from build123d import *

# Parameters (mm, degrees)
F0_W     = 62.186198
F0_H     = 153.296209
F1_DEPTH = 45.974
F2_R     = 22.70519
F3_DEPTH = 32.258
F5_DEPTH = 24.384


with BuildPart() as f1:
    # F0 (on Front) → F1 (new body)
    with BuildSketch(Plane.XZ):
        with Locations((1.59081, -0.433858)):
            Rectangle(F0_W, F0_H)
    extrude(amount=F1_DEPTH)

    # F2 (on face) → F3 (join)
    with BuildSketch(Plane.XZ.offset(45.974)):
        Circle(F2_R)
    extrude(amount=F3_DEPTH)

    # F4 (on Right) → F5 (cut, symmetric)
    with BuildSketch(Plane.YZ):
        Polygon((-53.611651, -25.310941), (-78.850865, 22.487216), (-78.627512, -25.310941), align=None)
    extrude(amount=F5_DEPTH, both=True, mode=Mode.SUBTRACT)


solid = f1.part
Build history of the part. All positions in model axes, mm. A direction names the side the tool comes from. Coordinates: 2 decimals unless noted, no trailing zeros. Order: outer loops, then holes, each group sorted by start corner. A loop starts at its lowest first (then second) coordinate and runs counter-clockwise, first axis right, second up. Notation, with made-up numbers: (-23.5, 18.25) - (-4.5, 18.25) arc R22 cw to (-4.5, 24.25) - close; hole circle Ø8 at (85, -38). An arc over 180 degrees is marked (long way). Write item = value, one per line. Start each with the question number.
1) Saw through at D-D on x = 26.5. Write the cut outline in (y, z), then the cut area to 3 significant figures.
2) Saw through at A-A on x = 0. Write the cut outline in (y, z).
3) 3-axis set-ups, long thin cutter, end or side, ignore diameter. For faces 1 (the face through (-2.96, -58.29, 22.51)), 2 (the face through (0.32, -66.45, -1)): which of +Z, -Z, +X, -X, +Y, -Y reach the whole face in a straight line?
4) Saw through at B-B on z = -1.5. Write the cut outline in (x, y), then the cut area to 3 significant figures.
5) Wall check: line 1 along Y through (x, z) = (9.5, 43); line 2 along X through (y, z) = (-53.5, 10.5); line 3 along Z through (x, y) = (4.5, -52.5). Give the ranges that are in metal, low to high. Write a range as from..to.
6) Flat gauge pins, fed straight in: pin 1 Ø4 at (x, y) = (-2.5, -65.5) entering from +Z; pin 2 Ø10 at (x, z) = (26, 38) entering from -Y; pin 3 Ø12 at (x, z) = (8, -6) entering from -Y. Where does each tip first touch, or does it go through?
7) Saw through at C-C on y = -49. Write the cut outline in (x, z), then the cut area to 3 significant figures.
From the geometry:
q1.outline = (-45.97, -77.08) - (0, -77.08) - (0, 76.21) - (-45.97, 76.21) - close
q1.area = 7,050 mm^2
q2.outline = (-78.23, 21.32) - (-54.99, -22.71) - (-45.97, -22.71) - (-45.97, -77.08) - (0, -77.08) - (0, 76.21) - (-45.97, 76.21) - (-45.97, 22.71) - (-78.23, 22.71) - close
q3.face_1 = -Y
q3.face_2 = -Z, +X, -X, -Y
q4.outline = (-29.5, -45.97) - (-22.66, -45.97) - (-22.66, -66.18) - (22.66, -66.18) - (22.66, -45.97) - (32.68, -45.97) - (32.68, 0) - (-29.5, 0) - close
q4.area = 3,770 mm^2
q5.line_1 = -45.97..0
q5.line_2 = -20.13..20.13
q5.line_3 = -22.25..22.25
q6.pin_1 = 22.7
q6.pin_2 = -45.97
q6.pin_3 = -66.98
q7.outline = circle Ø45.41 at (0, 0)
q7.area = 1,620 mm^2
